Build history of the part. All positions in model axes, mm. Give positions to 0.01 mm unless a question says otherwise; leave off trailing zeros. Loops run counter-clockwise (first coordinate to the right, second up) from the corner with the lowest first, then second, coordinate; pieces in that order, holes last. Notation, with made-up numbers: M 89.5,23 L 107.5,23 A20 ccw 107.5,36 Z; hole C -7.5,74.5 d3. An arc over 180 degrees is marked long. Answer as a JSON object with one key per item and string values. Group by question number.
1. Drop flat-ended pins along their axis: pin 1 Ø1.2 at (x, y) = (642, -1) entering from +Z; pin 2 Ø2 at (y, z) = (-2, 92.5) entering from -X; pin 3 Ø12 at (x, z) = (555, 311.5) entering from +Y; pin 4 Ø2 at (x, y) = (650, -1.5) entering from -Z. Give the stop position or say it passes through.
2. Slice it at D-D (y = -1.9). List the corners of the cut face in (x, z), then the cut area to 3 significant figures.
3. Slice it at B-B (z = 89). Give the number of separate pieces and of enclosed holes in the cut face, then the cut area to 3 significant figures.
4. Drill centre lines: line 1 along X through (y, z) = (-3.8, 158); line 2 along X through (y, z) = (-0.6, 283); line 3 along Z through (x, y) = (220, -3.6). Where is each one in solid material? Low to high. Write a range as [from, to].
from build123d import *

# Parameters (mm, degrees)
F0_W     = 115
F0_H     = 80.54
F0_W_2   = 434
F0_H_2   = 462.7
F1_DEPTH = 4
F2_SIZE  = 3.99999


# Not quite as in the source:
# - a fillet or chamfer is up to 0.001 mm smaller than in the source, because OpenCascade refuses the exact size


with BuildPart() as f1:
    # F0 (on Front) → F1 (new body)
    with BuildSketch(Plane.XZ):
        Polygon((0, 582.7), (0, 0), (509, 0), (559, 0), (758, 0), (758, 582.7), (559, 582.7), (509, 582.7), align=None)
        with Locations((631.5, 100.27)):
            Rectangle(F0_W, F0_H, mode=Mode.SUBTRACT)
        with Locations((631.5, 195.81)):
            Rectangle(F0_W, F0_H, mode=Mode.SUBTRACT)
        with Locations((282, 291.35)):
            Rectangle(F0_W_2, F0_H_2, mode=Mode.SUBTRACT)
        with Locations((631.5, 291.35)):
            Rectangle(F0_W, F0_H, mode=Mode.SUBTRACT)
        with Locations((631.5, 386.89)):
            Rectangle(F0_W, F0_H, mode=Mode.SUBTRACT)
        with Locations((631.5, 482.43)):
            Rectangle(F0_W, F0_H, mode=Mode.SUBTRACT)
    extrude(amount=F1_DEPTH)

    # F2 (size 4 in the source; OpenCascade refuses exactly that, so slightly less here)
    f2_edges = [f1.edges().sort_by_distance(p)[0] for p in [
        (379, 0, 0),
        (758, 0, 291.35),
        (0, 0, 291.35),
        (379, 0, 582.7),
    ]]
    chamfer(f2_edges, length=F2_SIZE)


solid = f1.part
Established:
{
 "1": {"pin 1": "stops at z = 580.3", "pin 2": "stops at x = 1", "pin 3": "stops at y = 0", "pin 4": "stops at z = 1.5"},
 "2": {"outline": "M 2.1,2.1 L 755.9,2.1 L 755.9,580.6 L 2.1,580.6 Z; hole M 65,60 L 499,60 L 499,522.7 L 65,522.7 Z; hole M 574,60 L 689,60 L 689,140.54 L 574,140.54 Z; hole M 574,155.54 L 689,155.54 L 689,236.08 L 574,236.08 Z; hole M 574,251.08 L 689,251.08 L 689,331.62 L 574,331.62 Z; hole M 574,346.62 L 689,346.62 L 689,427.16 L 574,427.16 Z; hole M 574,442.16 L 689,442.16 L 689,522.7 L 574,522.7 Z", "area": "189,000 mm^2"},
 "3": {"separate pieces": "3", "enclosed holes": "0", "area": "820 mm^2"},
 "4": {"line 1": "x = [0.2, 65], [499, 574], [689, 757.8]", "line 2": "x = [3.4, 65], [499, 574], [689, 754.6]", "line 3": "z = [0.4, 60], [522.7, 582.3]"}
}
